from build123d import *

# Parameters (mm, degrees)
F0_W     = 32
F0_H     = 10
F1_DEPTH = 25
F2_W     = 52
F2_H     = 10
F2_W_2   = 25
F3_DEPTH = 1


with BuildPart() as f1:
    # F0 (on Front) → F1 (new body)
    with BuildSketch(Plane.XZ):
        with Locations((-4.601419, 2.851491)):
            Rectangle(F0_W, F0_H)
    extrude(amount=F1_DEPTH)

    # F2 (on face) → F3 (join)
    with BuildSketch(Plane.YZ.offset(11.398581)):
        with Locations((-51, 2.851491)):
            Rectangle(F2_W, F2_H)
        with Locations((-12.5, 2.851491)):
            Rectangle(F2_W_2, F2_H)
    extrude(amount=F3_DEPTH)


solid = f1.part
Read the model definition and answer for the solid it produces. Units are mm, in the model's axes. A direction names the side the tool comes from. Give positions to 0.01 mm unless a question says otherwise; leave off trailing zeros. Write each loop counter-clockwise with the first axis right and the second up, starting at its lowest first coordinate (ties: lowest second). Pieces come first, ordered by that corner, then holes. Notation, with made-up numbers: (45.25, -37.75) - (89.25, -37.75) arc R22 ccw to (89.25, -3.75) - close; hole circle Ø6 at (9.25, -16.75). An arc over 180 degrees is marked (long way). Use CSV: the item, a comma, the result in double quotes. Start each with the question number.
Item 1: A flat-ended cylindrical pin translates along its axis: P1, Ø5, axis at x = -5, z = 4, coming from the -Y side. Find the tip coordinate at first contact, or state that the pin passes through.
Item 2: The part is cut by section A-A, the plane x = 6. Give the vertices of the cut face in (y, z).
Item 3: For faces 1 (the flat face through (-5, -25, 3)), 2 (the flat face through (-2, -16, 7.851)), determine the directions among +Z, -Z, +X, -X, +Y, -Y from which every point of the face is accessible in a straight line to the end or side of a thin tool.
Item 4: The part is cut by section C-C, the plane z = 5.5. Give the vertices of the cut face in (x, y), and give its area (3 significant figures).
Item 5: Consider line 1 (X direction, y = -52, z = 0); line 2 (Y direction, x = -6, z = 4.75). Determine where each line is inside the solid, lowest interval first.
Item 6: The part is cut by section B-B, the plane y = -42. Give the vertices of the cut face in (x, z).
Taken from the geometry:
1,P1,"y = -25"
2,outline,"(-25, -2.15) - (0, -2.15) - (0, 7.85) - (-25, 7.85) - close"
3,face 1,"+Z, -Z, -X, -Y"
3,face 2,"+Z, +X, -X, +Y, -Y"
4,outline,"(-20.6, -25) - (11.4, -25) - (11.4, -77) - (12.4, -77) - (12.4, 0) - (-20.6, 0) - close"
4,area,"877 mm2"
5,line 1,"11.4 to 12.4"
5,line 2,"-25 to 0"
6,outline,"(11.4, -2.15) - (12.4, -2.15) - (12.4, 7.85) - (11.4, 7.85) - close"
